from build123d import *

# Parameters (mm, degrees)
F0_R     = 5.08
F0_R_2   = 0.0254
F0_W     = 42.184448801
F0_H     = 73.8955140114
F0_R_3   = 2.1477431595
F1_DEPTH = 6.35


# Not quite as in the source:
# - ends of sketch curves that miss each other by under 0.0002 mm in the source are joined


with BuildPart() as f1:
    # F0 (on Front) → F1 (new body)
    with BuildSketch(Plane.XZ):
        with BuildLine():
            ThreePointArc((-55.3989668916, 62.6738528225), (-59.6104772855, 60.6747009039), (-61.3217708439, 56.3382389188))
            Line((-61.3217708439, 56.3382389188), (-61.3217708439, -32.5617610812))
            ThreePointArc((-61.3217708439, -32.5617610812), (-59.4618989044, -37.0518891418), (-54.9717708439, -38.9117610812))
            Line((-54.9717708439, -38.9117610812), (-16.8717708439, -38.9117610812))
            ThreePointArc((-16.8717708439, -38.9117610812), (-12.3816427833, -37.0518891418), (-10.5217708439, -32.5617610812))
            Line((-10.5217708439, -32.5617610812), (-10.5217708439, 56.3382389188))
            ThreePointArc((-10.5217708439, 56.3382389188), (-12.3824811709, 60.8292052103), (-16.8741419405, 62.6882384761))
            Line((-16.8741419405, 62.6882384761), (-55.3989668916, 62.6738528225))
        make_face()
        with Locations((-35.5558670086, -27.8927588342)):
            Circle(F0_R, mode=Mode.SUBTRACT)
        with Locations((-46.6527380049, 56.3382389188)):
            Circle(F0_R_2, mode=Mode.SUBTRACT)
        with Locations((-35.4520422406, 16.1202251911)):
            Rectangle(F0_W, F0_H, mode=Mode.SUBTRACT)
        with Locations((-35.2948196232, 58.1041015685)):
            Circle(F0_R_3, mode=Mode.SUBTRACT)
    extrude(amount=F1_DEPTH)


solid = f1.part
Build history of the part. All positions in model axes, mm. A direction names the side the tool comes from. Give positions to 0.01 mm unless a question says otherwise; leave off trailing zeros. Loops run counter-clockwise (first coordinate to the right, second up) from the corner with the lowest first, then second, coordinate; pieces in that order, holes last. Notation, with made-up numbers: (-22, 82) -> (-9, 82) arc R11 cw to (-9, 94) -> close; hole circle Ø10 at (-0.5, 70). An arc over 180 degrees is marked (long way). Answer in a Markdown table with one row per item.
Item 1: Tool access for faces 1 (the flat face through (-36, -3, -20.828)), 2 (the flat face through (-14, 0, 1)): list every direction of +Z, -Z, +X, -X, +Y, -Y with a clear straight run to the whole face (end or side of a thin tool).
Findings below:
| item | result |
|---|---|
| face 1 | +Y, -Y |
| face 2 | +Z, -Z, +X, -X, +Y |
Item 2: Mould opens along Z. For faces 3 (the flat face through (-61.322, -3, 13)), 4 (the cylindrical face through (-12.43, -3.13, -37.1)), 5 (the cylindrical face through (-12.333, -3.131, 60.78)), 6 (the flat face through (-36, -3, 53.068)) say: pulls with the +Z half, pulls with the -Z half, needs draft (parallel to the pull), parting line crosses it, or undercut.
Findings below:
| item | result |
|---|---|
| face 3 | needs draft |
| face 4 | pulls with the -Z half |
| face 5 | pulls with the +Z half |
| face 6 | undercut |
Item 3: Slice it at D-D on x = -39.5. Write the cut outline in (y, z).
Findings below:
| item | result |
|---|---|
| outline | (-6.35, -38.91) -> (0, -38.91) -> (0, -31.09) -> (-6.35, -31.09) -> close; (-6.35, -24.69) -> (0, -24.69) -> (0, -20.83) -> (-6.35, -20.83) -> close; (-6.35, 53.07) -> (0, 53.07) -> (0, 62.68) -> (-6.35, 62.68) -> close |
Item 4: Probe line 1 along Z through (x, y) = (-46, -1.75); line 2 along X through (y, z) = (-2.5, 31.5); line 3 along Z through (x, y) = (-35, -1.5). List the from-to ranges inside material, lowest first. Write a range as [from, to].
Findings below:
| item | result |
|---|---|
| line 1 | z = [-38.91, -20.83], [53.07, 62.68] |
| line 2 | x = [-61.32, -56.54], [-14.36, -10.52] |
| line 3 | z = [-38.91, -32.94], [-22.84, -20.83], [53.07, 55.98], [60.23, 62.68] |
Item 5: Slice it at B-B on x = -23.5. Write the cut outline in (y, z), plus the area to 3 significant figures.
Findings below:
| item | result |
|---|---|
| outline | (-6.35, -38.91) -> (0, -38.91) -> (0, -20.83) -> (-6.35, -20.83) -> close; (-6.35, 53.07) -> (0, 53.07) -> (0, 62.69) -> (-6.35, 62.69) -> close |
| area | 176 mm² |
Item 6: Slice it at C-C on y = -3.25. Write the cut outline in (x, z).
Findings below:
| item | result |
|---|---|
| outline | (-61.32, -32.56) arc R6.35 ccw to (-54.97, -38.91) -> (-16.87, -38.91) arc R6.35 ccw to (-10.52, -32.56) -> (-10.52, 56.34) arc R6.35 ccw to (-16.87, 62.69) -> (-55.4, 62.67) arc R6.35 ccw to (-61.32, 56.34) -> close; hole (-56.54, -20.83) -> (-14.36, -20.83) -> (-14.36, 53.07) -> (-56.54, 53.07) -> close; hole circle Ø0.05 at (-46.65, 56.34); hole circle Ø10.16 at (-35.56, -27.89); hole circle Ø4.3 at (-35.29, 58.1) |
Item 7: Slice it at A-A on z = -2. Write the cut outline in (x, y).
Findings below:
| item | result |
|---|---|
| outline | (-61.32, -6.35) -> (-56.54, -6.35) -> (-56.54, 0) -> (-61.32, 0) -> close; (-14.36, -6.35) -> (-10.52, -6.35) -> (-10.52, 0) -> (-14.36, 0) -> close |
